```python
from build123d import *

# Parameters (mm, degrees)
F0_W     = 38.1
F0_H     = 38.1
F1_DEPTH = 381
F2_T     = -3.175
F3_R     = 3.175


with BuildPart() as f1:
    # F0 (on Right) → F1 (new body)
    with BuildSketch(Plane.YZ):
        Rectangle(F0_W, F0_H)
    extrude(amount=F1_DEPTH)

    # F2
    f2_openings = [f1.faces().sort_by_distance(p)[0] for p in [
        (381, 0, 0),
        (0, 0, 0),
    ]]
    offset(amount=F2_T, openings=f2_openings)

    # F3
    f3_edges = [f1.edges().sort_by_distance(p)[0] for p in [
        (190.5, -19.05, 19.05),
        (190.5, 19.05, 19.05),
        (190.5, -19.05, -19.05),
        (190.5, 19.05, -19.05),
    ]]
    fillet(f3_edges, radius=F3_R)


solid = f1.part
```
Can you work these out from the model? Positions are in its coordinate system, mm. A direction names the side the tool comes from. Coordinates: 2 decimals unless noted, no trailing zeros. Write each loop counter-clockwise with the first axis right and the second up, starting at its lowest first coordinate (ties: lowest second). Pieces come first, ordered by that corner, then holes. Notation, with made-up numbers: M -7,11.25 L 43,11.25 A10 cw 43,19.25 Z; hole C -11,89 d4. An arc over 180 degrees is marked long. Write item = value, one per line. Start each with the question number.
Q1. On a 3-axis mill with a long thin cutter (end or side, diameter ignored), from which of +Z, -Z, +X, -X, +Y, -Y can I reach the whole of each face in a straight line? I mean faces 1 (the face through (188, 19.05, 0)), 2 (the face through (188, 0, 15.875)). Say none if no direction works.
Q2. Thinking about a two-plate mould opening in Z: for faces 3 (the face through (188, 15.875, 0)), 4 (the face through (188, -19.05, 0)), 5 (the face through (188, 0, 19.05)), which applies, released by +Z, released by -Z, zero draft, split by the parting line, or undercut?
Q3. If we section it at A-A, the plane z = 9: Write out the boundary of the cut face in (x, y) (3 decimals).
Q4. If we section it at B-B, the plane x = 174: Write out the boundary of the cut face in (y, z) (3 decimals), then the cut area to 3 significant figures.
Q5. If I drill on L1, parallel to Z at x = 142, y = 5.5 (3 decimals); L2, parallel to Y at x = 95, z = 16, over which ranges is the centre line in solid material (lowest first)? Write a range as [from, to].
Check sheet entries:
q1.face_1 = +Z, -Z, +X, -X, +Y
q1.face_2 = +X, -X
q2.face_3 = undercut
q2.face_4 = zero draft
q2.face_5 = released by +Z
q3.outline = M 0,-19.05 L 381,-19.05 L 381,-15.875 L 0,-15.875 Z; M 0,15.875 L 381,15.875 L 381,19.05 L 0,19.05 Z
q4.outline = M -19.05,-15.875 A3.175 ccw -15.875,-19.05 L 15.875,-19.05 A3.175 ccw 19.05,-15.875 L 19.05,15.875 A3.175 ccw 15.875,19.05 L -15.875,19.05 A3.175 ccw -19.05,15.875 Z; hole M -15.875,-15.875 L 15.875,-15.875 L 15.875,15.875 L -15.875,15.875 Z
q4.area = 435 mm²
q5.L1 = [-19.05, -15.875], [15.875, 19.05]
q5.L2 = [-19.05, 19.05]
